Here's the drawing with two shaded views (mm, measured from the low corner). I have some questions. Give positions to 0.01 mm unless a question says otherwise; leave off trailing zeros. Loops run counter-clockwise (first coordinate to the right, second up) from the corner with the lowest first, then second, coordinate; pieces in that order, holes last. Notation, with made-up numbers: (64, 74) - (68, 74) arc R19 cw to (68, 80) - close; hole circle Ø11 at (7, -10). An arc over 180 degrees is marked (long way). Write each question's results on one line, items separated by ' | '. Start each with the question number.
1) I want a section at B-B, the plane y = 0.6. Write out the boundary of the cut face in (x, z).
2) I'm going to push a flat-ended pin straight in: pin 1 (2 mm diameter, centred on x = 7.5, z = 13.5, fed in from +Y). Where does the tip first touch, or does it pass through?
3) If I drill on probe 1 along Z at (x, y) = (45, 1.3); probe 2 along Z at (x, y) = (22, 0.4); probe 3 along X at (y, z) = (0.6, 12.5), over which ranges is the centre line in solid material (lowest first)? Write a range as [from, to].
4) I want a section at D-D, the plane x = 33. Write out the boundary of the cut face in (y, z).
5) I want a section at A-A, the plane z = 4.5. Write out the boundary of the cut face in (x, y).
6) I want a section at C-C, the plane x = 76.5. Write out the boundary of the cut face in (y, z), and give its area (3 significant figures).
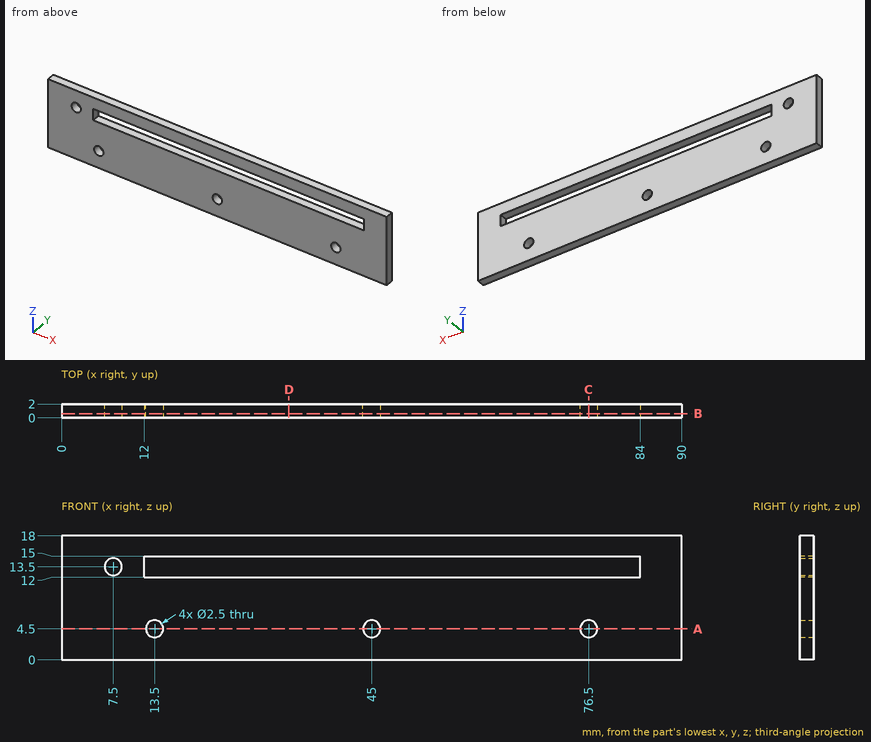
Answers:
1) outline: (0, 0) - (90, 0) - (90, 18) - (0, 18) - close; hole circle Ø2.5 at (7.5, 13.5); hole (12, 12) - (84, 12) - (84, 15) - (12, 15) - close; hole circle Ø2.5 at (13.5, 4.5); hole circle Ø2.5 at (45, 4.5); hole circle Ø2.5 at (76.5, 4.5)
2) pin 1: passes through
3) probe 1: z = [0, 3.25], [5.75, 12], [15, 18] | probe 2: z = [0, 12], [15, 18] | probe 3: x = [0, 6.75], [8.25, 12], [84, 90]
4) outline: (0, 0) - (2, 0) - (2, 12) - (0, 12) - close; (0, 15) - (2, 15) - (2, 18) - (0, 18) - close
5) outline: (0, 0) - (12.25, 0) - (12.25, 2) - (0, 2) - close; (14.75, 0) - (43.75, 0) - (43.75, 2) - (14.75, 2) - close; (46.25, 0) - (75.25, 0) - (75.25, 2) - (46.25, 2) - close; (77.75, 0) - (90, 0) - (90, 2) - (77.75, 2) - close
6) outline: (0, 0) - (2, 0) - (2, 3.25) - (0, 3.25) - close; (0, 5.75) - (2, 5.75) - (2, 12) - (0, 12) - close; (0, 15) - (2, 15) - (2, 18) - (0, 18) - close | area: 25.0 mm2
